For this review, take the finished solid that the model builds, in its own axes (mm). Face numbers are marked on the shaded views. A direction names the side the tool comes from. Round coordinates to 2 decimals unless told otherwise and drop trailing zeros. Write each loop counter-clockwise with the first axis right and the second up, starting at its lowest first coordinate (ties: lowest second). Pieces come first, ordered by that corner, then holes. Notation, with made-up numbers: (-27, 67.25) -> (5, 67.25) arc R28 cw to (5, 85.25) -> close; hole circle Ø9 at (-4, -7.75). An arc over 180 degrees is marked (long way). Answer as CSV lines item,"result". Start each with the question number.
Item 1: Machinability: for the marked faces 4 and 5, which of the approach directions +Z, -Z, +X, -X, +Y, -Y give a long, thin tool a straight path to every point of the face, cutting with its end or side? Answer none if there is none.
Item 2: For pin 1 Ø10 at (x, z) = (-1, 29.5) entering from -Y; pin 2 Ø4 at (x, z) = (18.5, 28.5) entering from +Y, all flat-tipped, find the tip position at first contact; note any pin that passes through.
Item 3: Take a section at A-A on y = 17. Count the separate pieces of the cut face and the enclosed holes in it, then the cut area to 3 significant figures.
Item 4: Mouldability with a two-part tool opening along Y and no side actions: class the marked faces 1, 2 and 3 as +Y half, -Y half, draft (parallel to the pull), parting line (faces both ways), or undercut.
Item 5: Take a section at C-C on y = -5. Give the boundary of the cut face in (x, z), then the cut area to 3 significant figures.
Item 6: Wall thickness on probe 1 along Z at (x, y) = (19, 20.7) (1 decimal); probe 2 along X at (y, z) = (-15, 13.5); probe 3 along X at (y, z) = (0, 21.5) (3 decimals): over which ranges is each line inside the solid? List them lowest first. Write a range as from..to.
```python
from build123d import *
from build123d.topology import SkipClean

# Parameters (mm, degrees)
EXTRUSION1_DEPTH = 36.869499995
THREAD6_D        = 5.25
THREAD6_DEPTH    = 20
THREAD6_TIP      = 1.577259125
THREAD10_D       = 5.25
THREAD10_DEPTH   = 17
SKETCH6_W        = 48
SKETCH6_H        = 36.869499995
SKETCH6_R        = 2.625
EXTRUSION2_DEPTH = 1.869499995
CHAMFER2_SIZE    = 0.5


with BuildPart() as part:
    # Sketch1 → Extrusion1 (new body)
    with BuildSketch(Plane.XY):
        with BuildLine():
            Line((-24, 20), (24, 20))
            Line((24, 20), (24, -20))
            Line((24, -20), (8.5, -20))
            Line((8.5, -20), (8.5, -11.187157816))
            ThreePointArc((8.5, -11.187157816), (0, 14.05), (-8.5, -11.187157816))
            Line((-8.5, -11.187157816), (-8.5, -20))
            Line((-8.5, -20), (-24, -20))
            Line((-24, -20), (-24, 20))
        make_face()
    extrude(amount=EXTRUSION1_DEPTH)

    # Thread6
    with Locations(Plane.XY.offset(36.869499995)):
        with Locations((-19, 0), (-13.435028843, -13.435028843), (-13.435028843, 13.435028843), (13.435028843, 13.435028843), (19, 0), (13.435028843, -13.435028843)):
            Hole(THREAD6_D / 2, depth=THREAD6_DEPTH)
            with Locations((0, 0, -(THREAD6_DEPTH + THREAD6_TIP / 2))):  # 118° drill point
                Cone(0, THREAD6_D / 2, THREAD6_TIP, mode=Mode.SUBTRACT)

    # Thread10
    with Locations(Plane(origin=(0, 20, 0), x_dir=(1, 0, 0), z_dir=(0, 1, 0))):
        with Locations((-19, -6.5), (19, -6.5), (-19, -28.5), (19, -28.5)):
            Hole(THREAD10_D / 2, depth=THREAD10_DEPTH)

    # Sketch6 → Extrusion2 (add)
    with SkipClean():  # the faces are left unmerged after this step: merging them gives an invalid solid
        with BuildSketch(Plane(origin=(0, 20, 0), x_dir=(-1, 0, 0), z_dir=(0, 1, 0))):
            with Locations((0, 18.434749998)):
                Rectangle(SKETCH6_W, SKETCH6_H)
            with Locations(Location((19, 28.5, 0), (0, 0, 90))):
                Circle(SKETCH6_R, mode=Mode.SUBTRACT)
            with Locations(Location((19, 6.5, 0), (0, 0, 90))):
                Circle(SKETCH6_R, mode=Mode.SUBTRACT)
            with Locations(Location((-19, 6.5, 0), (0, 0, 90))):
                Circle(SKETCH6_R, mode=Mode.SUBTRACT)
            with Locations(Location((-19, 28.5, 0), (0, 0, 90))):
                Circle(SKETCH6_R, mode=Mode.SUBTRACT)
        extrude(amount=EXTRUSION2_DEPTH)

    # Chamfer2
    chamfer2_edges = [part.edges().sort_by_distance(p)[0] for p in [
        (24, 21.869499995, 18.434749997),
        (0, 21.869499995, 0),
        (-24, 21.869499995, 18.434749997),
    ]]
    chamfer(chamfer2_edges, length=CHAMFER2_SIZE)


solid = part.part
```
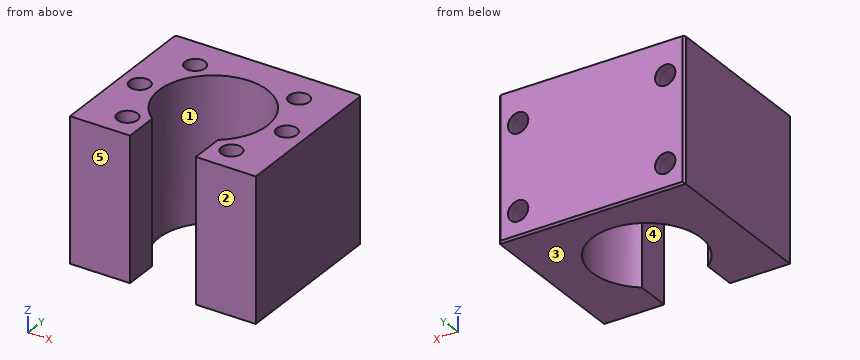
Output values:
1,face 4,"+Z, -Z, -Y"
1,face 5,"+Z, -Z, +X, -X, -Y"
2,pin 1,"stops at y = 12.7"
2,pin 2,"stops at y = 3"
3,separate pieces,"1"
3,enclosed holes,"4"
3,area,"1,680 mm^2"
4,face 1,"undercut"
4,face 2,"-Y half"
4,face 3,"draft"
5,outline,"(-24, 0) -> (-13.13, 0) -> (-13.13, 36.87) -> (-24, 36.87) -> close; (13.13, 0) -> (24, 0) -> (24, 36.87) -> (13.13, 36.87) -> close"
5,area,"802 mm^2"
6,probe 1,"z = 0..3.9, 9.1..25.9, 31.1..36.9"
6,probe 2,"x = -24..-8.5, 8.5..24"
6,probe 3,"x = -24..-21.625, -16.375..-14.05, 14.05..16.375, 21.625..24"
